Drawing for the job (mm, zero at the part's lowest x, y, z). Coordinates: 2 decimals unless noted, no trailing zeros. Loops run counter-clockwise (first coordinate to the right, second up) from the corner with the lowest first, then second, coordinate; pieces in that order, holes last. Notation, with made-up numbers: (-22, 56.5) -> (30, 56.5) arc R14 ccw to (30, 66.5) -> close; hole circle Ø9 at (-12, 34.25). An arc over 180 degrees is marked (long way). Write item = value, one per line. Start each with the question number.
(1) Band-saw the part on A-A (x = 38). Write the cut outline in (y, z) (1 decimal).
(2) Band-saw the part on D-D (x = 15.24). Write the cut outline in (y, z) (1 decimal).
(3) Flat gauge pins, fed straight in: P1, Ø1.6, axis at y = 1, z = 54, coming from the +X side; P2, Ø1.5, axis at y = 2, z = 83.5, coming from the -X side (1 decimal). Where does each tip first touch, or does it go through?
(4) Drill centre lines: line 1 (Z direction, x = 36, y = 2.8) (1 decimal); line 2 (X direction, y = 1, z = 67.5) (1 decimal); line 3 (X direction, y = 1.9, z = 35). Where is each one in solid material? Low to high. Write a range as from..to.
(5) Band-saw the part on B-B (z = 6.35). Count the separate pieces of the cut face and the enclosed holes in it.
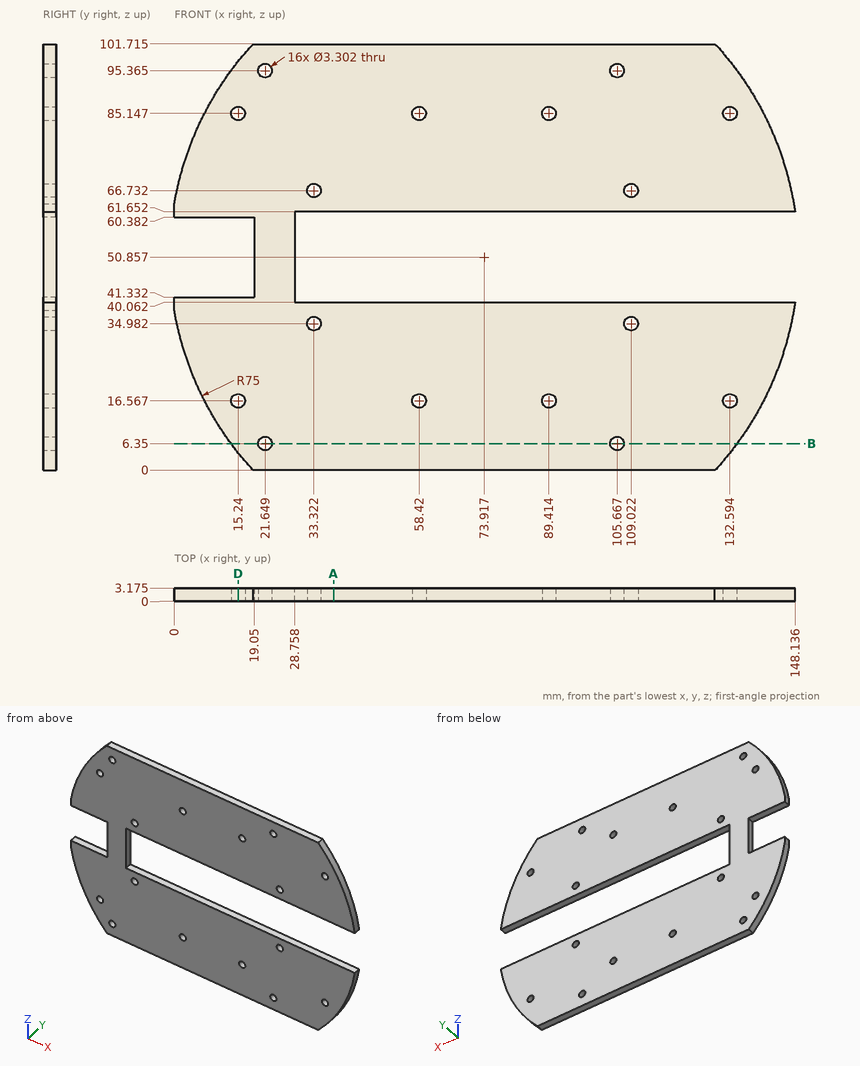
Findings below:
q1.outline = (0, 0) -> (3.2, 0) -> (3.2, 40.1) -> (0, 40.1) -> close; (0, 61.7) -> (3.2, 61.7) -> (3.2, 101.7) -> (0, 101.7) -> close
q2.outline = (0, 4.1) -> (3.2, 4.1) -> (3.2, 14.9) -> (0, 14.9) -> close; (0, 18.2) -> (3.2, 18.2) -> (3.2, 41.3) -> (0, 41.3) -> close; (0, 60.4) -> (3.2, 60.4) -> (3.2, 83.5) -> (0, 83.5) -> close; (0, 86.8) -> (3.2, 86.8) -> (3.2, 97.6) -> (0, 97.6) -> close
q3.P1 = 28.76
q3.P2 = 6
q4.line_1 = 0..40.1, 61.7..101.7
q4.line_2 = 0.8..31.9, 34.8..107.6, 110.5..147
q4.line_3 = 0.61..31.67, 34.97..107.37, 110.67..147.22
q5.separate_pieces = 3
q5.enclosed_holes = 0
